Geometry: see drawing. Coordinates: mm, zero at the bounding-box minimum. A direction names the side the tool comes from. Round coordinates to 2 decimals unless told otherwise and drop trailing zeros. Loops run counter-clockwise (first coordinate to the right, second up) from the corner with the lowest first, then second, coordinate; pieces in that order, holes last.
(1) Cut plane C-C, the plane x = 103.5. Output: boundary loops of the cut face in (y, z), and give its area (3 significant figures).
(2) Line query: line 1 (Y direction, x = 375, z = 3); line 2 (Z direction, x = 119, y = 25.5); line 3 (X direction, y = 24.5, z = 7) (1 decimal). Output: solid intervals per line, ascending.
(3) Cut plane B-B, the plane z = 25. Give the number of separate pieces and of enclosed holes in the cut face, and give its area (3 significant figures).
(4) Draft query along X for the marked faces 1 and 2. Return one class per face: released by +X, released by -X, zero draft, split by the parting line, or undercut.
(5) Access query for the marked faces 3 and 4. Directions: +Z, -Z, +X, -X, +Y, -Y. A direction counts if a zero-diameter tool reaches every point of the face in a straight line with its end or side. Return the directions, or none.
(6) First-contact query: pin 1 Ø1 at (y, z) = (20, 2.5) entering from -X; pin 2 Ø8 at (y, z) = (25.5, 26) entering from +X; pin 3 Ø9.5 at (x, y) = (59.5, 13) entering from -Z (3 decimals). Flat tips, straight axial feed; report the tip coordinate or a pass-through.
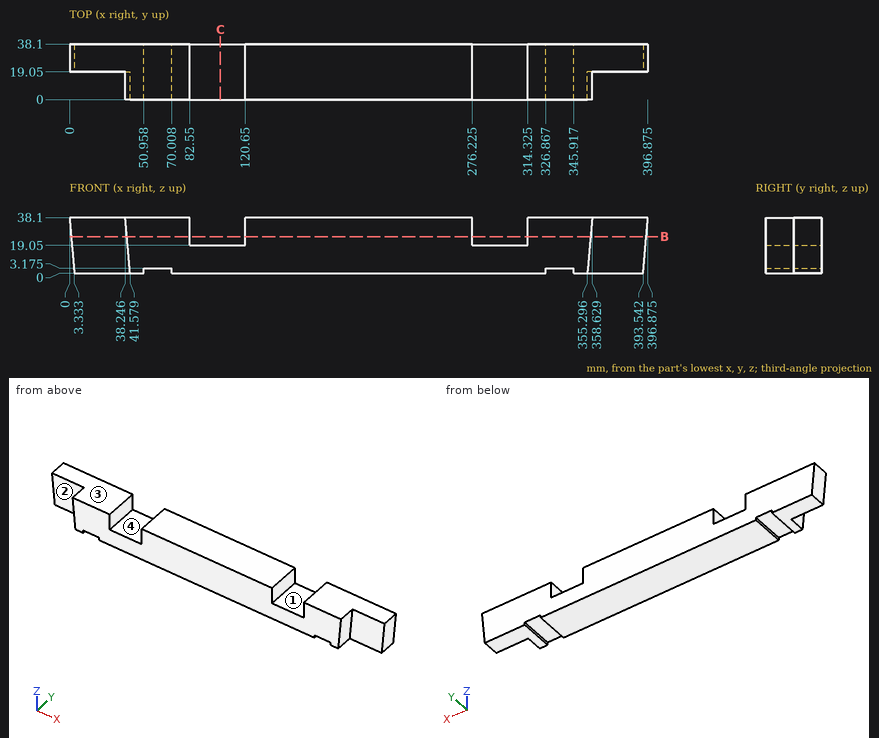
Reported:
1. outline: (0, 0) - (38.1, 0) - (38.1, 19.05) - (0, 19.05) - close
1. area: 726 mm2
2. line 1: y = 19.05 to 38.1
2. line 2: z = 0 to 19.05
2. line 3: x = 2.7 to 394.2
3. separate pieces: 3
3. enclosed holes: 0
3. area: 10,700 mm2
4. face 1: undercut
4. face 2: zero draft
5. face 3: +Z, +X, -X, +Y, -Y
5. face 4: +Z, +Y, -Y
6. pin 1: stops at x = 3.07
6. pin 2: stops at x = 396.17
6. pin 3: stops at z = 3.175
